from build123d import *

# Parameters (mm, degrees)
F0_W     = 914.4
F0_H     = 2133.6
F4_DEPTH = 76.2
F6_D     = 101.6
F7_D     = 25.4
F8_DEPTH = 25.4
F2_W     = 152.4
F2_H     = 381
F9_DEPTH = 25.4


with BuildPart() as f4:
    # F0 (on Front) → F4 (new body)
    with BuildSketch(Plane.XZ):
        with Locations((457.2, 1066.8)):
            Rectangle(F0_W, F0_H)
    extrude(amount=F4_DEPTH)

    # F6 (through all)
    with Locations(Plane(origin=(0, 0, 0), x_dir=(1, 0, 0), z_dir=(0, 1, 0))):
        with Locations((799.4753718376, -1064.6243095398)):
            Hole(F6_D / 2)

    # F7 (through all)
    with Locations(Plane.XZ.offset(76.2)):
        with Locations((452.9111683369, 1495.7164525986)):
            Hole(F7_D / 2)

    # F1 (on Front) → F8 (cut)
    with BuildSketch(Plane.XZ):
        with BuildLine():
            ThreePointArc((787.4, 1708.7225914001), (457.2, 2038.9225914001), (127, 1708.7225914001))
            Line((127, 1708.7225914001), (787.4, 1708.7225914001))
        make_face()
    extrude(amount=F8_DEPTH, mode=Mode.SUBTRACT)

    # F2 (on Front) → F9 (cut)
    with BuildSketch(Plane.XZ):
        with Locations((331.3514550252, 907.5841558799)):
            Rectangle(F2_W, F2_H)
        with Locations((636.1514550252, 907.5841558799)):
            Rectangle(F2_W, F2_H)
        with Locations((331.3514550252, 399.5841558799)):
            Rectangle(F2_W, F2_H)
        with Locations((626.4034242401, 399.9588191742)):
            Rectangle(F2_W, F2_H)
    extrude(amount=F9_DEPTH, mode=Mode.SUBTRACT)


solid = f4.part
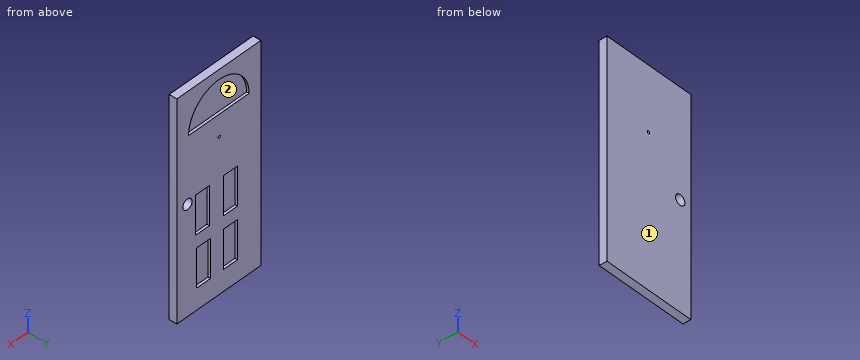
Read the model definition and answer for the solid it produces. Units are mm, in the model's axes. Face numbers are marked on the shaded views. Coordinates: 2 decimals unless noted, no trailing zeros. Loops run counter-clockwise (first coordinate to the right, second up) from the corner with the lowest first, then second, coordinate; pieces in that order, holes last. Notation, with made-up numbers: (-22, 59) - (-10, 59) arc R12 cw to (-10, 66) - close; hole circle Ø11 at (24.5, 22.25). An arc over 180 degrees is marked (long way). Answer in a Markdown table with one row per item.
Q1. Straight lines are drawn through the part: line 1 along X through (y, z) = (-7.5, 930); line 2 along X through (y, z) = (-14, 263); line 3 along Y through (x, z) = (389.5, 1895). For each, find the intervals that lie inside material, in ascending order. Write a range as [from, to].
Here are the results:
| item | result |
|---|---|
| line 1 | x = [0, 255.15], [407.55, 559.95], [712.35, 914.4] |
| line 2 | x = [0, 255.15], [407.55, 550.2], [702.6, 914.4] |
| line 3 | y = [-76.2, -25.4] |
Q2. Find section A-A on z = 235. Write down the section's boundary in (x, y).
Here are the results:
| item | result |
|---|---|
| outline | (0, -76.2) - (914.4, -76.2) - (914.4, 0) - (702.6, 0) - (702.6, -25.4) - (550.2, -25.4) - (550.2, 0) - (407.55, 0) - (407.55, -25.4) - (255.15, -25.4) - (255.15, 0) - (0, 0) - close |
Q3. The mould has two halves that part along X. Classify the marked faces 1 and 2: pulls with the +X half, pulls with the -X half, needs draft (parallel to the pull), parting line crosses it, or undercut.
Here are the results:
| item | result |
|---|---|
| face 1 | needs draft |
| face 2 | undercut |
Q4. Find section C-C on z = 1973.5. Write down the section's boundary in (x, y).
Here are the results:
| item | result |
|---|---|
| outline | (0, -76.2) - (914.4, -76.2) - (914.4, 0) - (654.49, 0) - (654.49, -25.4) - (259.91, -25.4) - (259.91, 0) - (0, 0) - close |
Q5. Find section B-B on x = 647. Write down the section's boundary in (y, z), plus the area to 3 significant figures.
Here are the results:
| item | result |
|---|---|
| outline | (-76.2, 0) - (0, 0) - (0, 209.46) - (-25.4, 209.46) - (-25.4, 590.46) - (0, 590.46) - (0, 717.08) - (-25.4, 717.08) - (-25.4, 1098.08) - (0, 1098.08) - (0, 1708.72) - (-25.4, 1708.72) - (-25.4, 1978.92) - (0, 1978.92) - (0, 2133.6) - (-76.2, 2133.6) - close |
| area | 136,000 mm^2 |
Q6. Given P1, Ø10, axis at x = 381, z = 913, coming from the +Y side; P2, Ø15, axis at x = 452.91, z = 1495.72, coming from the -Y side, each flat-ended and moving along its own axis, determine where each tip first touches the part or whether it passes through.
Here are the results:
| item | result |
|---|---|
| P1 | stops at y = -25.4 |
| P2 | passes through |
